Study the drawing (mm; zero at the part's minimum x, y, z) and answer. A direction names the side the tool comes from. Coordinates: 2 decimals unless noted, no trailing zeros. Order: outer loops, then holes, each group sorted by start corner. A loop starts at its lowest first (then second) coordinate and runs counter-clockwise, first axis right, second up.
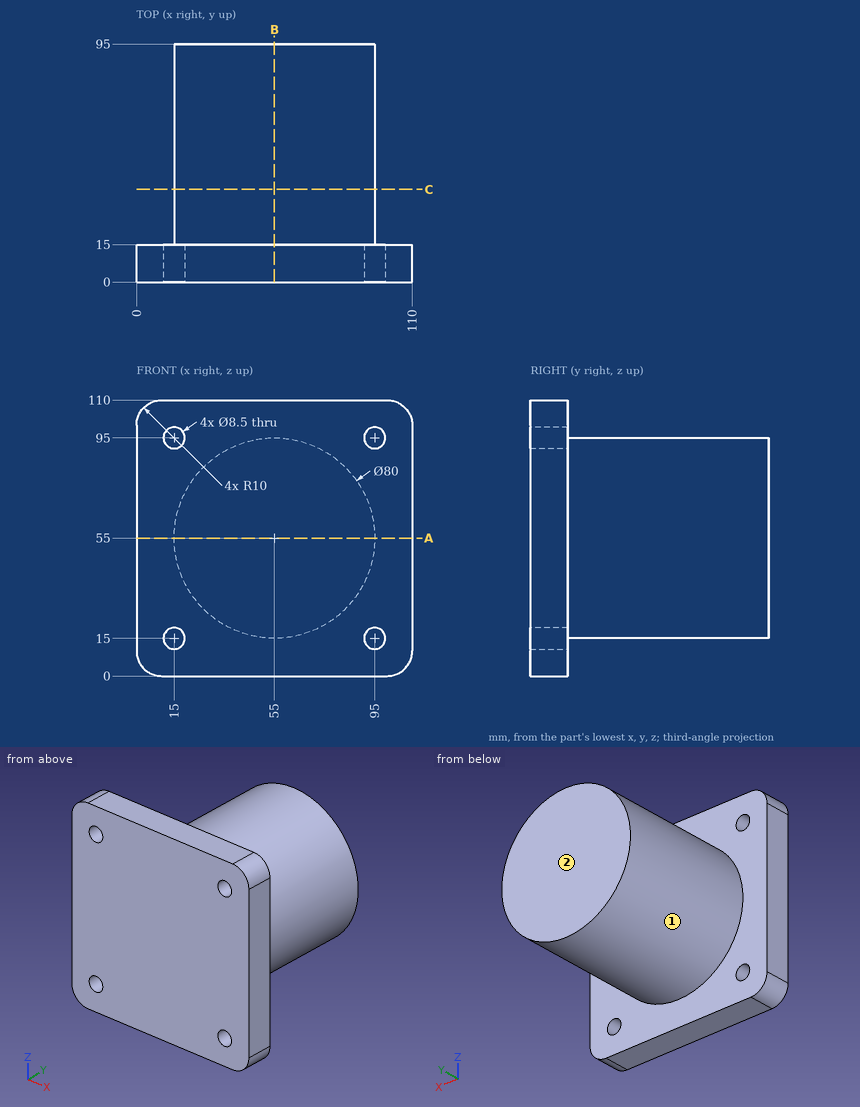
1) A cutting plane is placed at C-C, the plane y = 37. Determine the outline of the cut face in (x, z).
A:
outline: circle Ø80 at (55, 55)
2) A cutting plane is placed at B-B, the plane x = 55. Determine the outline of the cut face in (y, z).
A:
outline: (0, 0) - (15, 0) - (15, 15) - (95, 15) - (95, 95) - (15, 95) - (15, 110) - (0, 110) - close
3) Flat-ended cylindrical pins translate along their axes: pin 1 Ø12 at (y, z) = (35.5, 15.5) entering from -X; pin 2 Ø12 at (y, z) = (60, 29) entering from -X; pin 3 Ø3 at (x, y) = (59.5, 55.5) entering from -Z; pin 4 Ø7 at (x, z) = (95, 95) entering from +Y. Find the tip coordinate at first contact, or state that the pin passes through.
A:
pin 1: stops at x = 33.14
pin 2: stops at x = 20.36
pin 3: stops at z = 15.11
pin 4: passes through
4) A cutting plane is placed at A-A, the plane z = 55. Determine the outline of the cut face in (x, y).
A:
outline: (0, 0) - (110, 0) - (110, 15) - (95, 15) - (95, 95) - (15, 95) - (15, 15) - (0, 15) - close
5) Which of the six approach directions +Z, -Z, +X, -X, +Y, -Y give full straight-line access (tool end or side, diameter ignored) to the marked faces 1 and 2?
A:
face 1: +Y
face 2: +Z, -Z, +X, -X, +Y
6) Straight lines are drawn through the part: line 1 (X direction, y = 5, z = 15); line 2 (Y direction, x = 85, z = 15); line 3 (X direction, y = 9.5, z = 97). For each, find the intervals that lie inside material, in ascending order.
A:
line 1: x = 0 to 10.75, 19.25 to 90.75, 99.25 to 110
line 2: y = 0 to 15
line 3: x = 0 to 11.25, 18.75 to 91.25, 98.75 to 110
